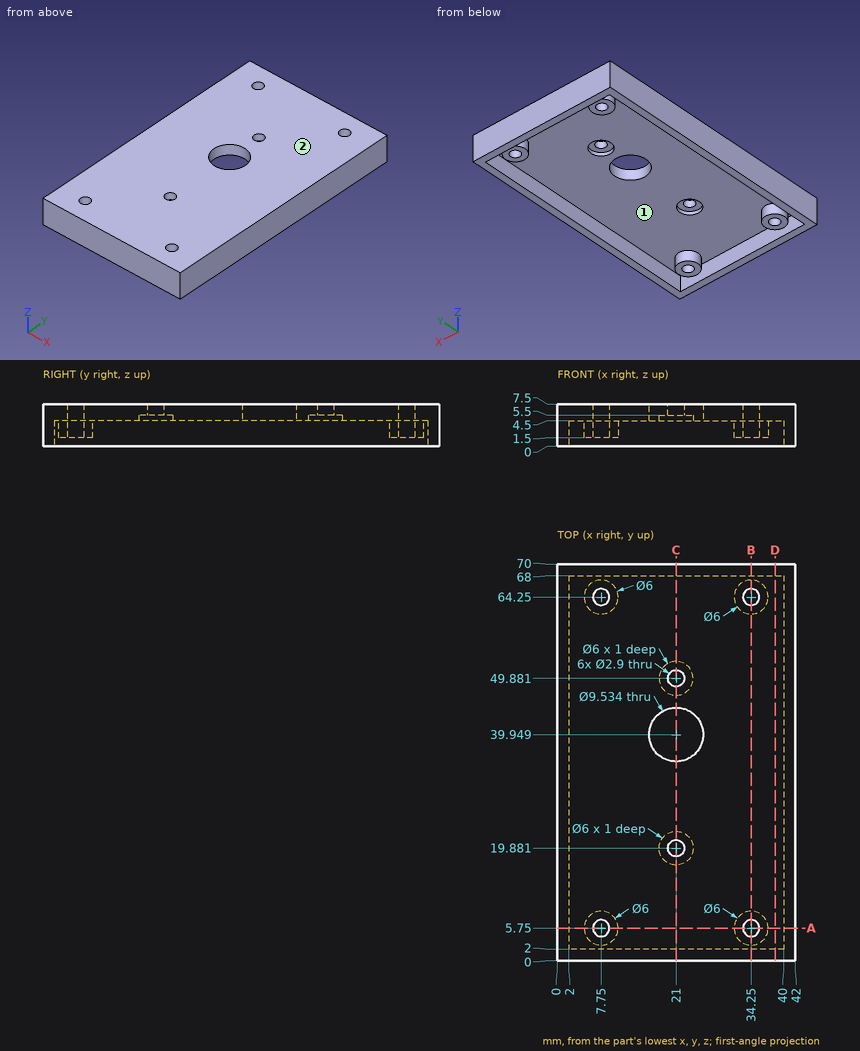
For this review, use the dimensioned drawing (mm, ordinates from the lowest corner) and the shaded views. A direction names the side the tool comes from. Give positions to 0.01 mm unless a question says otherwise; leave off trailing zeros. Loops run counter-clockwise (first coordinate to the right, second up) from the corner with the lowest first, then second, coordinate; pieces in that order, holes last.
Item 1: Take a section at B-B, the plane x = 34.25. State the section outline as (y, z) points, and give its area (3 significant figures).
Item 2: Take a section at A-A, the plane y = 5.75. State the section outline as (x, z) points, and give its area (3 significant figures).
Item 3: For line 1 along Y through (x, z) = (21, 6.6); line 2 along Y through (x, z) = (21, 4.75); line 3 along Y through (x, z) = (4, 3.5), list the stretches that pass through material, from the lowest coordinate up.
Item 4: Tool access review of the marked faces 1 and 2: name each direction out of +Z, -Z, +X, -X, +Y, -Y from which nothing blocks a thin tool from reaching the whole face with its end or side.
Item 5: Insertion check: pin 1 (10 mm diameter, centred on x = 24, y = 27.5, fed in from -Z); pin 2 (3 mm diameter, centred on y = 18, z = 5, fed in from -X); pin 3 (5.5 mm diameter, centred on x = 21, y = 49.88, fed in from -Z); pin 4 (3 mm diameter, centred on x = 33.5, y = 65.5, fed in from -Z). Each pin has a flat end and moves straight along its axis. Give the tip position at first contact, or say it passes through.
Item 6: Take a section at C-C, the plane x = 21. State the section outline as (y, z) points, and give its area (3 significant figures).
Item 7: Take a section at D-D, the plane x = 38.5. State the section outline as (y, z) points.
Calculated:
1. outline: (0, 0) - (2, 0) - (2, 4.5) - (2.75, 4.5) - (2.75, 1.5) - (4.3, 1.5) - (4.3, 7.5) - (0, 7.5) - close; (7.2, 1.5) - (8.75, 1.5) - (8.75, 4.5) - (61.25, 4.5) - (61.25, 1.5) - (62.8, 1.5) - (62.8, 7.5) - (7.2, 7.5) - close; (65.7, 1.5) - (67.25, 1.5) - (67.25, 4.5) - (68, 4.5) - (68, 0) - (70, 0) - (70, 7.5) - (65.7, 7.5) - close
1. area: 229 mm2
2. outline: (0, 0) - (2, 0) - (2, 4.5) - (4.75, 4.5) - (4.75, 1.5) - (6.3, 1.5) - (6.3, 7.5) - (0, 7.5) - close; (9.2, 1.5) - (10.75, 1.5) - (10.75, 4.5) - (31.25, 4.5) - (31.25, 1.5) - (32.8, 1.5) - (32.8, 7.5) - (9.2, 7.5) - close; (35.7, 1.5) - (37.25, 1.5) - (37.25, 4.5) - (40, 4.5) - (40, 0) - (42, 0) - (42, 7.5) - (35.7, 7.5) - close
2. area: 145 mm2
3. line 1: y = 0 to 18.43, 21.33 to 35.18, 44.72 to 48.43, 51.33 to 70
3. line 2: y = 0 to 16.88, 22.88 to 35.18, 44.72 to 46.88, 52.88 to 70
3. line 3: y = 0 to 2, 68 to 70
4. face 1: -Z
4. face 2: +Z, +X, -X, +Y, -Y
5. pin 1: stops at z = 4.5
5. pin 2: stops at x = 0
5. pin 3: stops at z = 5.5
5. pin 4: stops at z = 1.5
6. outline: (0, 0) - (2, 0) - (2, 4.5) - (16.88, 4.5) - (16.88, 5.5) - (18.43, 5.5) - (18.43, 7.5) - (0, 7.5) - close; (21.33, 5.5) - (22.88, 5.5) - (22.88, 4.5) - (35.18, 4.5) - (35.18, 7.5) - (21.33, 7.5) - close; (44.72, 4.5) - (46.88, 4.5) - (46.88, 5.5) - (48.43, 5.5) - (48.43, 7.5) - (44.72, 7.5) - close; (51.33, 5.5) - (52.88, 5.5) - (52.88, 4.5) - (68, 4.5) - (68, 0) - (70, 0) - (70, 7.5) - (51.33, 7.5) - close
6. area: 176 mm2
7. outline: (0, 0) - (2, 0) - (2, 4.5) - (68, 4.5) - (68, 0) - (70, 0) - (70, 7.5) - (0, 7.5) - close
